```python
from build123d import *

# Parameters (mm, degrees)
F1_DEPTH = 10
F2_R     = 7.5
F3_DEPTH = 7.5
F3_TAPER = 45
F4_R     = 7.5


# Not quite as in the source:
# - an extrude whose draft closes it to a point is written as a loft to that point


with BuildPart() as f1:
    # F0 (on Top) → F1 (new body)
    with BuildSketch(Plane.XY):
        with BuildLine():
            Line((51.71875, 3.3977172854), (-28.28125, 3.3977172854))
            ThreePointArc((-28.28125, 3.3977172854), (-43.28125, -11.6022827146), (-28.28125, -26.6022827146))
            Line((-28.28125, -26.6022827146), (51.71875, -26.6022827146))
            ThreePointArc((51.71875, -26.6022827146), (66.71875, -11.6022827146), (51.71875, 3.3977172854))
        make_face()
    extrude(amount=F1_DEPTH)

    # F2 (on face) → F3 (join)
    with BuildSketch(Plane.XY.offset(10)):
        with Locations((-28.28125, -11.6022827146)):
            Circle(F2_R)
    extrude(amount=F3_DEPTH, taper=F3_TAPER)

    # F4 (on face) → F5 section 0
    with BuildSketch(Plane(origin=(0, 0, 0), x_dir=(1, 0, 0), z_dir=(0, 0, -1)), mode=Mode.PRIVATE) as f5_s0:
        with Locations((51.71875, 11.6022827146)):
            Circle(F4_R)
    loft([f5_s0.sketch, Vertex(51.71875, -11.6022827146, 7.5)], ruled=True, mode=Mode.SUBTRACT)


solid = f1.part
```
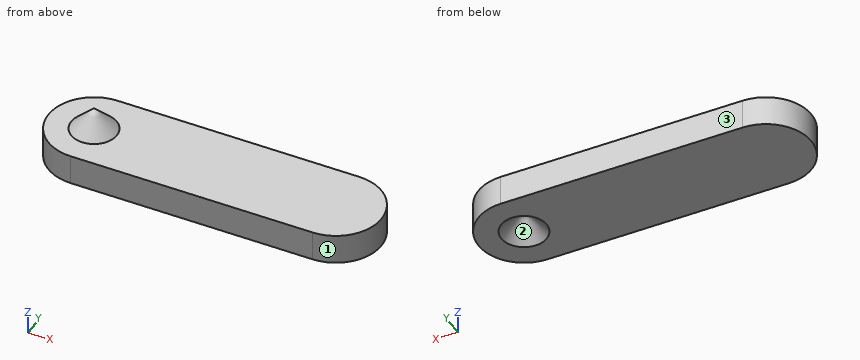
Read the model definition and answer for the solid it produces. Units are mm, in the model's axes. Face numbers are marked on the shaded views. Coordinates: 2 decimals unless noted, no trailing zeros. Write each loop counter-clockwise with the first axis right and the second up, starting at its lowest first coordinate (ties: lowest second). Pieces come first, ordered by that corner, then holes. Notation, with made-up numbers: (79.5, 36) -> (128.5, 36) arc R19 ccw to (128.5, 45) -> close; hole circle Ø5 at (59.25, 58). An arc over 180 degrees is marked (long way). Write item = value, one per line.
(1) Section A-A on z = 6 is taken. Write down the section's boundary in (x, y), plus the area to 3 significant figures.
From the geometry:
outline = (-28.28, -26.6) -> (51.72, -26.6) arc R15 ccw to (51.72, 3.4) -> (-28.28, 3.4) arc R15 ccw to start; hole circle Ø3 at (51.72, -11.6)
area = 3,100 mm2
(2) Section B-B on x = 18.5 is taken. Write down the section's boundary in (y, z).
From the geometry:
outline = (-26.6, 0) -> (3.4, 0) -> (3.4, 10) -> (-26.6, 10) -> close
(3) For a pull along X with two mould halves and no side action, classify the marked faces 1, 2 and 3 as +X half, -X half, draft (parallel to the pull), parting line (faces both ways), or undercut.
From the geometry:
face_1 = +X half
face_2 = undercut
face_3 = draft
(4) Section D-D on z = 14.25 is taken. Write down the section's boundary in (x, y), plus the area to 3 significant figures.
From the geometry:
outline = circle Ø6.5 at (-28.28, -11.6)
area = 33.2 mm2
(5) Straight lines are drawn through the part: L1, parallel to Z at x = -4, y = -4.75; L2, parallel to X at y = -15.25, z = 2.5; L3, parallel to X at y = -3.5, z = 7.25. For each, find the intervals that lie inside material, in ascending order. Write a range as from..to.
From the geometry:
L1 = 0..10
L2 = -42.83..48.3, 55.14..66.27
L3 = -40.9..64.34
(6) Section C-C on y = -2.5 is taken. Write down the section's boundary in (x, z).
From the geometry:
outline = (-40.2, 0) -> (63.64, 0) -> (63.64, 10) -> (-40.2, 10) -> close
(7) Given pin 1 Ø6 at (y, z) = (-23, 8) entering from +X; pin 2 Ø10 at (x, y) = (41, -6) entering from +Z; pin 3 Ø1 at (x, y) = (-8.5, 0) entering from -Z, each flat-ended and moving along its own axis, determine where each tip first touches the part or whether it passes through.
From the geometry:
pin_1 = 64.15
pin_2 = 10
pin_3 = 0
